Geometry check sheet. Reference: the model listing, model coordinates, mm. Face numbers are marked on the shaded views. Coordinates: 2 decimals unless noted, no trailing zeros. Loops run counter-clockwise (first coordinate to the right, second up) from the corner with the lowest first, then second, coordinate; pieces in that order, holes last. Notation, with made-up numbers: (-25, -13) -> (19, -13) arc R9 cw to (19, 1) -> close; hole circle Ø7 at (9.25, 89.5). An arc over 180 degrees is marked (long way). Answer as a JSON object with one key per item and string values.
from build123d import *

# Parameters (mm, degrees)
BOSS_EXTRUDE1_DEPTH = 4
SKETCH2_R           = 2
CUT_EXTRUDE1_DEPTH  = 29.296371725
SKETCH3_R           = 13.5
BOSS_EXTRUDE2_DEPTH = 3
SKETCH4_R           = 4
CUT_EXTRUDE2_DEPTH  = 29.87359785


with BuildPart() as part:
    # Sketch1 → Boss-Extrude1 (new body)
    with BuildSketch(Plane(origin=(0, 0, 0), x_dir=(1, 0, 0), z_dir=(0, 1, 0))):
        with BuildLine():
            ThreePointArc((13.5, 0), (13.159823391, 3.011486067), (12.156437284, 5.871203671))
            ThreePointArc((12.156437284, 5.871203671), (0, 13.5), (-12.156437284, 5.871203671))
            ThreePointArc((-12.156437284, 5.871203671), (-13.159823391, 3.011486067), (-13.5, 0))
            Line((-13.5, 0), (13.5, 0))
        make_face()
        with BuildLine():
            ThreePointArc((12.156437284, -5.871203671), (13.159823391, -3.011486067), (13.5, 0))
            Line((13.5, 0), (-13.5, 0))
            ThreePointArc((-13.5, 0), (-13.159823391, -3.011486067), (-12.156437284, -5.871203671))
            ThreePointArc((-12.156437284, -5.871203671), (0, -13.5), (12.156437284, -5.871203671))
        make_face()
        with BuildLine():
            ThreePointArc((-12.156437284, 5.871203671), (0, 13.5), (12.156437284, 5.871203671))
            Line((12.156437284, 5.871203671), (4.502384179, 21.719064136))
            ThreePointArc((4.502384179, 21.719064136), (0, 24.544544258), (-4.502384179, 21.719064136))
            Line((-4.502384179, 21.719064136), (-12.156437284, 5.871203671))
        make_face()
        with BuildLine():
            Line((4.502384179, -21.719064136), (12.156437284, -5.871203671))
            ThreePointArc((12.156437284, -5.871203671), (0, -13.5), (-12.156437284, -5.871203671))
            Line((-12.156437284, -5.871203671), (-4.502384179, -21.719064136))
            ThreePointArc((-4.502384179, -21.719064136), (0, -24.544544258), (4.502384179, -21.719064136))
        make_face()
    extrude(amount=BOSS_EXTRUDE1_DEPTH)

    # Sketch2 → Cut-Extrude1 (cut, through all)
    with BuildSketch(Plane(origin=(0, 4, 0), x_dir=(1, 0, 0), z_dir=(0, 1, 0))):
        with Locations(Location((0, -18, 0), (0, 0, 270))):
            Circle(SKETCH2_R)
        with Locations(Location((0, 18, 0), (0, 0, 270))):
            Circle(SKETCH2_R)
    extrude(amount=-CUT_EXTRUDE1_DEPTH, mode=Mode.SUBTRACT)

    # Sketch3 → Boss-Extrude2 (add)
    with BuildSketch(Plane(origin=(0, 4, 0), x_dir=(1, 0, 0), z_dir=(0, 1, 0))):
        with Locations(Location((0, 0, 0), (0, 0, 25.779183858))):
            Circle(SKETCH3_R)
    extrude(amount=BOSS_EXTRUDE2_DEPTH)

    # Sketch4 → Cut-Extrude2 (cut, through all)
    with BuildSketch(Plane(origin=(0, 7, 0), x_dir=(1, 0, 0), z_dir=(0, 1, 0))):
        with Locations(Location((0, 0, 0), (0, 0, 270))):
            Circle(SKETCH4_R)
    extrude(amount=-CUT_EXTRUDE2_DEPTH, mode=Mode.SUBTRACT)


solid = part.part
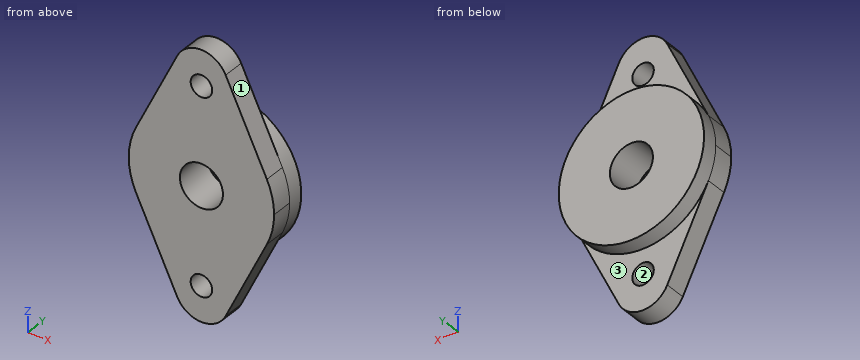
1. Section check D-D, the plane x = 3.25. Record the boundary of the cut face in (y, z), then the cut area to 3 significant figures.
Evaluation:
{"outline": "(0, -23.34) -> (4, -23.34) -> (4, -13.1) -> (7, -13.1) -> (7, -2.33) -> (0, -2.33) -> close; (0, 2.33) -> (7, 2.33) -> (7, 13.1) -> (4, 13.1) -> (4, 23.34) -> (0, 23.34) -> close", "area": "233 mm^2"}
2. Thickness scan on probe 1 along X at (y, z) = (5.75, 0); probe 2 along Z at (x, y) = (0.75, 1.5); probe 3 along Y at (x, z) = (-5.25, 18.5). Record the ranges inside material, lowest first. Write a range as from..to.
Evaluation:
{"probe 1": "x = -13.5..-4, 4..13.5", "probe 2": "z = -24.49..-19.85, -16.15..-3.93, 3.93..16.15, 19.85..24.49", "probe 3": "y = 0..4"}
3. Section check B-B, the plane z = 18. Record the boundary of the cut face in (x, y).
Evaluation:
{"outline": "(-6.3, 0) -> (-2, 0) -> (-2, 4) -> (-6.3, 4) -> close; (2, 0) -> (6.3, 0) -> (6.3, 4) -> (2, 4) -> close"}
4. Mould release check, pull along Z, two halves, no side actions. Record for the marked faces 1, 2 and 3: released by +Z, released by -Z, zero draft, split by the parting line, or undercut.
Evaluation:
{"face 1": "released by +Z", "face 2": "undercut", "face 3": "zero draft"}
5. Section check C-C, the plane y = 1.5. Record the boundary of the cut face in (x, z).
Evaluation:
{"outline": "(-12.16, -5.87) -> (-4.5, -21.72) arc R5 ccw to (4.5, -21.72) -> (12.16, -5.87) arc R13.5 ccw to (12.16, 5.87) -> (4.5, 21.72) arc R5 ccw to (-4.5, 21.72) -> (-12.16, 5.87) arc R13.5 ccw to start; hole circle Ø8 at (0, 0); hole circle Ø4 at (0, -18); hole circle Ø4 at (0, 18)"}
6. Depth check by flat-ended pin: P1, Ø3, axis at x = -5.5, y = 2, coming from the +Z side; P2, Ø2, axis at y = 1, z = 11, coming from the -X side; P3, Ø2, axis at y = 5.5, z = -8, coming from the -X side. Enter the tip coordinate at first touch or a pass-through.
Evaluation:
{"P1": "stops at z = 22.54", "P2": "stops at x = -10.16", "P3": "stops at x = -11.54"}
7. Section check A-A, the plane x = 0. Record the boundary of the cut face in (y, z), then the cut area to 3 significant figures.
Evaluation:
{"outline": "(0, -24.54) -> (4, -24.54) -> (4, -20) -> (0, -20) -> close; (0, -16) -> (4, -16) -> (4, -13.5) -> (7, -13.5) -> (7, -4) -> (0, -4) -> close; (0, 4) -> (7, 4) -> (7, 13.5) -> (4, 13.5) -> (4, 16) -> (0, 16) -> close; (0, 20) -> (4, 20) -> (4, 24.54) -> (0, 24.54) -> close", "area": "189 mm^2"}
